Geometry check sheet. Reference: the model listing, model coordinates, mm. Round coordinates to 2 decimals unless told otherwise and drop trailing zeros. Order: outer loops, then holes, each group sorted by start corner. A loop starts at its lowest first (then second) coordinate and runs counter-clockwise, first axis right, second up. Notation, with made-up numbers: (40, -10) -> (90, -10) arc R29 cw to (90, 10) -> close; hole circle Ø3 at (-9, -32.75). An arc over 180 degrees is marked (long way). Use a Markdown table: item, result. Add a question column.
Item 1: Gauge pin test, flat ends, axial feed: pin 1 Ø2 at (x, y) = (6, -35) entering from +Z; pin 2 Ø12 at (x, y) = (16.5, -28) entering from +Z; pin 3 Ø2.5 at (y, z) = (0, 0) entering from +X; pin 4 Ø12 at (x, y) = (33.5, 10.5) entering from +Z. Record the tip position at first contact, or that the pin passes through.
Item 2: Sectioned sample at D-D, the plane y = -21. Record the cut outline in (x, z), and give its area (3 significant figures).
Item 3: Material ranges on probe 1 along Y at (x, z) = (24, 0); probe 2 along Y at (x, z) = (4.5, -0.75); probe 3 along Z at (x, y) = (12.5, -32.5), recorded low to high. Write a range as [from, to].
Item 4: Sectioned sample at C-C, the plane y = -31. Record the cut outline in (x, z), and give its area (3 significant figures).
Item 5: Mould release check, pull along Z, two halves, no side actions. Record for faces 1 (the cylindrical face through (18.734, 23.333, -0.033)), 2 (the cylindrical face through (18.73, -22.91, -2.71)), 3 (the cylindrical face through (18.734, 0.631, -2.003)): pulls with the +Z half, pulls with the -Z half, needs draft (parallel to the pull), parting line crosses it, or undercut.
Item 6: Sectioned sample at B-B, the plane x = 20.5. Record the cut outline in (y, z).
Item 7: Sectioned sample at A-A, the plane z = 0. Record the cut outline in (x, y), and give its area (3 significant figures).
from build123d import *

# Parameters (mm, degrees)
SKETCH1_R           = 2.1
BOSS_EXTRUDE1_DEPTH = 38


with BuildPart() as part:
    # Sketch1 → Boss-Extrude1 (new body)
    with BuildSketch(Plane.YZ):
        with BuildLine():
            ThreePointArc((-45.166666667, 1.5), (-46.666666667, 0), (-45.166666667, -1.5))
            ThreePointArc((-45.166666667, -1.5), (-22.593289689, -2.724847701), (0, -3.5))
            ThreePointArc((0, -3.5), (10.925062805, -2.59165784), (21.833333333, -1.5))
            ThreePointArc((21.833333333, -1.5), (23.333333333, 0), (21.833333333, 1.5))
            ThreePointArc((21.833333333, 1.5), (10.925062805, 2.59165784), (0, 3.5))
            ThreePointArc((0, 3.5), (-22.593289689, 2.724847701), (-45.166666667, 1.5))
        make_face()
        with Locations(Location((0, 0, 0), (0, 0, 270))):
            Circle(SKETCH1_R, mode=Mode.SUBTRACT)
    extrude(amount=BOSS_EXTRUDE1_DEPTH)


solid = part.part
Found:
| question | item | result |
|---|---|---|
| 1 | pin 1 | stops at z = 2.16 |
| 1 | pin 2 | stops at z = 2.75 |
| 1 | pin 3 | passes through |
| 1 | pin 4 | stops at z = 3.15 |
| 2 | outline | (0, -2.79) -> (38, -2.79) -> (38, 2.79) -> (0, 2.79) -> close |
| 2 | area | 212 mm2 |
| 3 | probe 1 | y = [-46.67, -2.1], [2.1, 23.33] |
| 3 | probe 2 | y = [-46.47, -1.96], [1.96, 23.13] |
| 3 | probe 3 | z = [-2.24, 2.24] |
| 4 | outline | (0, -2.32) -> (38, -2.32) -> (38, 2.32) -> (0, 2.32) -> close |
| 4 | area | 176 mm2 |
| 5 | face 1 | parting line crosses it |
| 5 | face 2 | pulls with the -Z half |
| 5 | face 3 | undercut |
| 6 | outline | (-45.17, -1.5) arc R1135.34 ccw to (0, -3.5) arc R652.87 ccw to (21.83, -1.5) arc R1.5 ccw to (21.83, 1.5) arc R652.87 ccw to (0, 3.5) arc R1135.34 ccw to (-45.17, 1.5) arc R1.5 ccw to start; hole circle Ø4.2 at (0, 0) |
| 7 | outline | (0, -46.67) -> (38, -46.67) -> (38, -2.1) -> (0, -2.1) -> close; (0, 2.1) -> (38, 2.1) -> (38, 23.33) -> (0, 23.33) -> close |
| 7 | area | 2,500 mm2 |
